Read the model definition and answer for the solid it produces. Units are mm, in the model's axes. Face numbers are marked on the shaded views. Give positions to 0.01 mm unless a question says otherwise; leave off trailing zeros. Write each question's results on one line, items separated by ' | '. Start each with the question number.
Q1. Find section A-A on y = -28. Count the separate pieces of the cut face and the enclosed holes in it, and give its area (3 significant figures).
Q2. Find the intervals of material crossed by line 1 along X through (y, z) = (-27, -3.75); line 2 along X through (y, z) = (-26, -0.75); line 3 along X through (y, z) = (48, -1.25), in increasing order. Write a range as from..to.
Q3. Flat-ended cylindrical pins translate along their axes: P1, Ø1, axis at x = 53.5, z = -3, coming from the -Y side; P2, Ø4, axis at y = -24, z = -6, coming from the +X side; P3, Ø1, axis at x = 0, z = -3, coming from the +Y side; P4, Ø12, axis at x = -16, y = 16, coming from the +Z side. Find the tip coordinate at first contact, or state that the pin passes through.
Q4. For a pull along Z with two mould halves and no side action, classify the marked faces 1 and 2 as +Z half, -Z half, draft (parallel to the pull), parting line (faces both ways), or undercut.
from build123d import *

# Parameters (mm, degrees)
F0_R     = 17.7226640642
F0_R_2   = 18.3749948005
F0_R_3   = 17.2587936306
F0_R_4   = 17.3107234895
F1_DEPTH = 7
F1_TAPER = -3


with BuildPart() as f1:
    # F0 (on Top) → F1 (new body)
    with BuildSketch(Plane.XY):
        with BuildLine():
            Line((20.9337220527, 9.4692130681), (19.499204162, 41.8922447345))
            ThreePointArc((19.499204162, 41.8922447345), (0.4136393699, 69.3604386191), (-19.7564966048, 42.6784957835))
            Line((-19.7564966048, 42.6784957835), (-20.6694687182, 10.0329346663))
            Line((-20.6694687182, 10.0329346663), (-54.6471718869, -20.9214688483))
            ThreePointArc((-54.6471718869, -20.9214688483), (-60.7466147764, -57.9726414688), (-24.6403292313, -47.6610586484))
            Line((-24.6403292313, -47.6610586484), (-9.6195229838, -47.6610586484))
            Line((-9.6195229838, -47.6610586484), (-3.4192691352, -22.7199320794))
            Line((-3.4192691352, -22.7199320794), (2.290364122, -47.6610586484))
            Line((2.290364122, -47.6610586484), (7.1764700115, -22.7199320794))
            Line((7.1764700115, -22.7199320794), (13.8948652893, -47.6610586484))
            Line((13.8948652893, -47.6610586484), (27.5816481614, -47.6610586484))
            ThreePointArc((27.5816481614, -47.6610586484), (62.1265489826, -59.4900511481), (56.3092509412, -23.4423843748))
            Line((56.3092509412, -23.4423843748), (20.9337220527, 9.4692130681))
        make_face()
        with Locations((-45.9599420428, -41.3792170584)):
            Circle(F0_R, mode=Mode.SUBTRACT)
        Circle(F0_R_2, mode=Mode.SUBTRACT)
        with Locations((48.4029948711, -43.211504817)):
            Circle(F0_R_3, mode=Mode.SUBTRACT)
        with Locations((0, 48.7083792686)):
            Circle(F0_R_4, mode=Mode.SUBTRACT)
        Circle(F0_R_2)
        with Locations((48.4029948711, -43.211504817)):
            Circle(F0_R_3)
        with Locations((-45.9599420428, -41.3792170584)):
            Circle(F0_R)
    extrude(amount=-F1_DEPTH, taper=F1_TAPER)


solid = f1.part
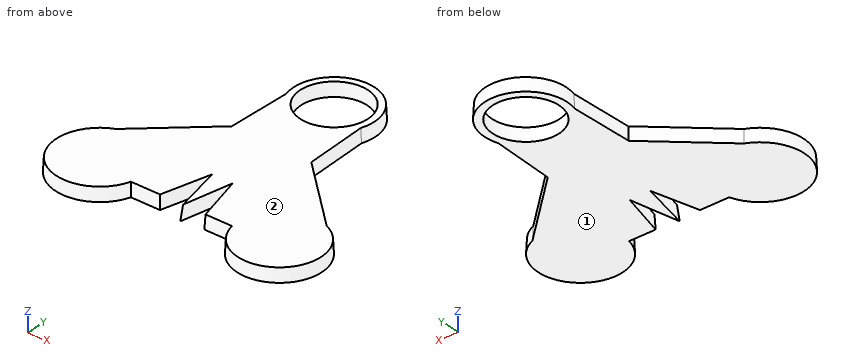
Working result:
1) separate pieces: 3 | enclosed holes: 0 | area: 863 mm²
2) line 1: -63.16..-4.28, -2.64..6.54, 8.13..62.51 | line 2: -62.06..-4.19, -2.71..6.57, 8.02..61 | line 3: -20.71..-17.23, 17.23..20.71
3) P1: y = -64.16 | P2: x = 61.47 | P3: y = 69.55 | P4: z = 0
4) face 1: -Z half | face 2: +Z half
